Drawing for the job (mm, zero at the part's lowest x, y, z). A direction names the side the tool comes from. Give positions to 0.01 mm unless a question says otherwise; leave off trailing zeros. Order: outer loops, then holes, each group sorted by start corner. A loop starts at its lowest first (then second) coordinate and runs counter-clockwise, first axis right, second up. Notation, with made-up numbers: (56, 47.5) -> (115, 47.5) arc R20 cw to (115, 65.5) -> close; hole circle Ø11 at (-31.75, 86). An arc over 180 degrees is marked (long way). One line per item, written item: value. Start each with the question number.
(1) Saw through at A-A on y = 9.25. Give the cut face in (x, z), plus the area to 3 significant figures.
(2) Two-plate mould, pull along Z, no slides. Class the marked faces 1, 2, 3 and 4: +Z half, -Z half, draft (parallel to the pull), parting line (faces both ways), or undercut.
(3) Saw through at B-B on z = 8. Give the cut face in (x, y), plus the area to 3 significant figures.
(4) Which spindle directions (+Z, -Z, +X, -X, +Y, -Y) get a long thin tool onto all of the face, cutting with end or side? Do the marked faces 5, 6 and 7. Say none if no direction does.
(5) Saw through at C-C on x = 17. Give the cut face in (y, z).
(6) Probe line 1 (X direction, y = 8, z = 8); line 2 (Z direction, x = 9, y = 5); line 3 (X direction, y = 7, z = 6). List the from-to ranges inside material, lowest first.
(7) Saw through at D-D on x = 3. Give the cut face in (y, z).
(8) Pin check, flat tips, straight feed: pin 1 (1.8 mm diameter, centred on x = 72, z = 22.5, fed in from +Y); pin 2 (2.5 mm diameter, centred on y = 1, z = 13, fed in from -X); pin 3 (1 mm diameter, centred on x = 32, z = 13.5, fed in from +Y). Stop position of each tip, or through.
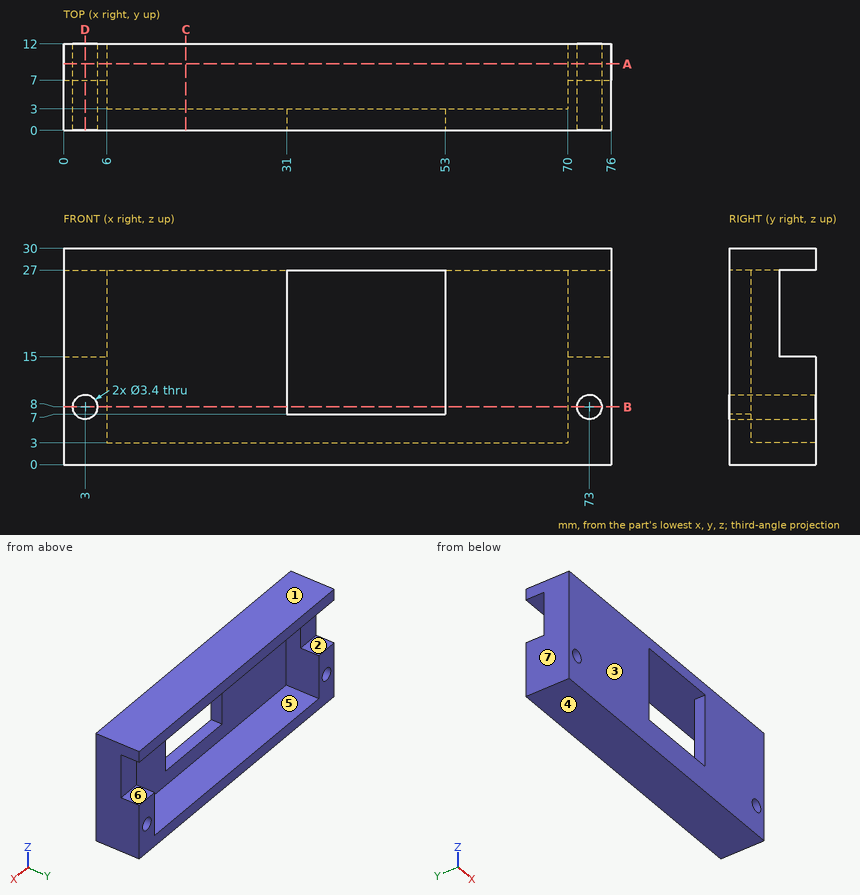
Results below:
1. outline: (0, 0) -> (76, 0) -> (76, 15) -> (70, 15) -> (70, 3) -> (6, 3) -> (6, 15) -> (0, 15) -> close; (0, 27) -> (76, 27) -> (76, 30) -> (0, 30) -> close; hole circle Ø3.4 at (3, 8); hole circle Ø3.4 at (73, 8)
1. area: 582 mm²
2. face 1: +Z half
2. face 2: undercut
2. face 3: draft
2. face 4: -Z half
3. outline: (0, 0) -> (1.3, 0) -> (1.3, 12) -> (0, 12) -> close; (4.7, 0) -> (31, 0) -> (31, 3) -> (6, 3) -> (6, 12) -> (4.7, 12) -> close; (53, 0) -> (71.3, 0) -> (71.3, 12) -> (70, 12) -> (70, 3) -> (53, 3) -> close; (74.7, 0) -> (76, 0) -> (76, 12) -> (74.7, 12) -> close
3. area: 188 mm²
4. face 5: +Y
4. face 6: +X, -X, +Y
4. face 7: +Z, -Z, -X, +Y, -Y
5. outline: (0, 0) -> (12, 0) -> (12, 3) -> (3, 3) -> (3, 27) -> (12, 27) -> (12, 30) -> (0, 30) -> close
6. line 1: x = 0 to 1.3, 4.7 to 6, 70 to 71.3, 74.7 to 76
6. line 2: z = 0 to 3, 27 to 30
6. line 3: x = 0 to 6, 70 to 76
7. outline: (0, 0) -> (12, 0) -> (12, 6.3) -> (0, 6.3) -> close; (0, 9.7) -> (12, 9.7) -> (12, 15) -> (7, 15) -> (7, 27) -> (12, 27) -> (12, 30) -> (0, 30) -> close
8. pin 1: stops at y = 7
8. pin 2: stops at x = 0
8. pin 3: passes through
